Print and shaded views of the part. All mm, measured from the part's lowest x, y and z. Coordinates: 2 decimals unless noted, no trailing zeros. Loops run counter-clockwise (first coordinate to the right, second up) from the corner with the lowest first, then second, coordinate; pieces in that order, holes last.
1) Two-plate mould, pull along X, no slides. Class the marked faces 1, 2 and 3: +X half, -X half, draft (parallel to the pull), parting line (faces both ways), or undercut.
2) Saw through at C-C, the plane y = 5.25. Write the cut outline in (x, z), and give its area (3 significant figures).
3) Saw through at B-B, the plane x = 44. Write the cut outline in (y, z).
4) Wall check: line 1 along X through (y, z) = (8, 44); line 2 along X through (y, z) = (6.75, 62.5) (1 decimal); line 3 along X through (y, z) = (0.5, 25). Give the ranges that are in metal, low to high.
5) Pin check, flat tips, straight feed: pin 1 Ø3 at (y, z) = (6.5, 48) entering from -X; pin 2 Ø2.5 at (x, z) = (76.04, 62.5) entering from +Y; pin 3 Ø4 at (x, z) = (12.5, 14) entering from -Y; pin 4 Ø4 at (y, z) = (9.5, 66.5) entering from +X. Stop position of each tip, or through.
6) Saw through at D-D, the plane z = 62.5. Write the cut outline in (x, y).
7) Saw through at A-A, the plane z = 44. Write the cut outline in (x, y).
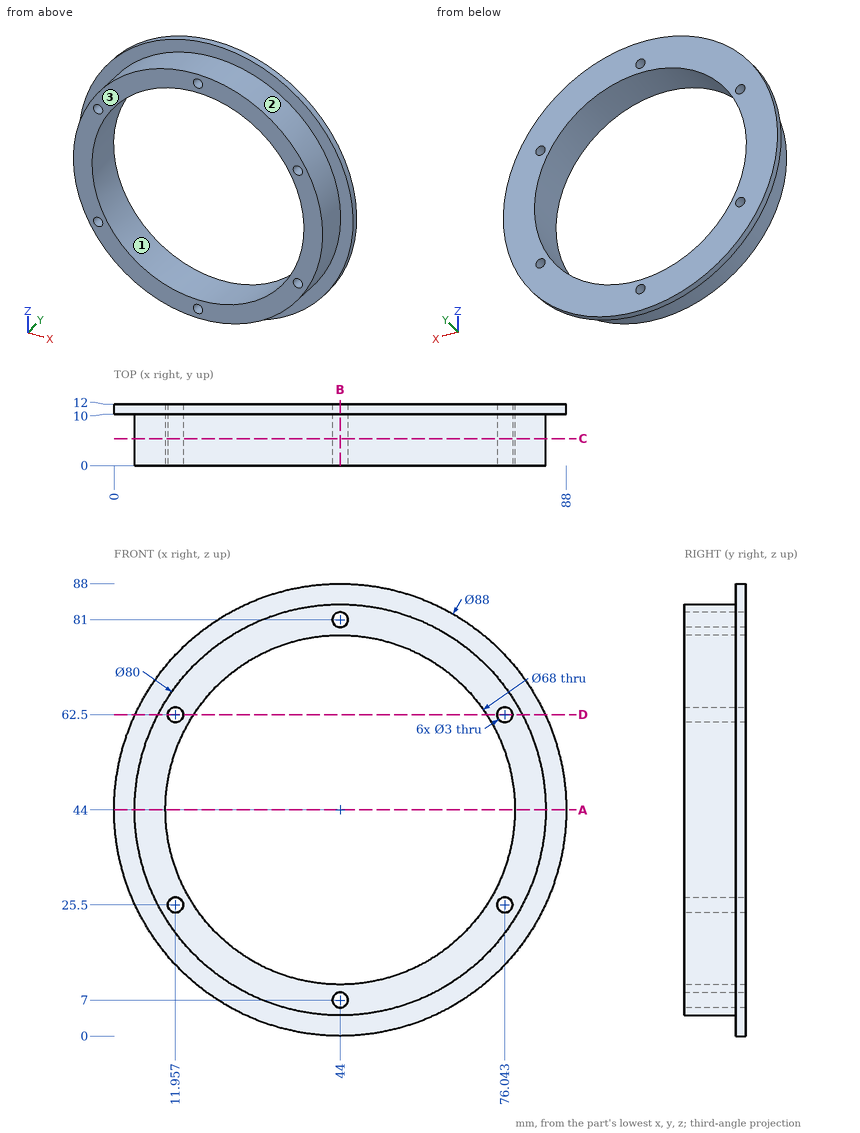
Data:
1. face 1: undercut
1. face 2: parting line
1. face 3: draft
2. outline: circle Ø80 at (44, 44); hole circle Ø68 at (44, 44); hole circle Ø3 at (11.96, 25.5); hole circle Ø3 at (11.96, 62.5); hole circle Ø3 at (44, 7); hole circle Ø3 at (44, 81); hole circle Ø3 at (76.04, 25.5); hole circle Ø3 at (76.04, 62.5)
2. area: 1,350 mm2
3. outline: (0, 4) - (10, 4) - (10, 0) - (12, 0) - (12, 5.5) - (0, 5.5) - close; (0, 8.5) - (12, 8.5) - (12, 10) - (0, 10) - close; (0, 78) - (12, 78) - (12, 79.5) - (0, 79.5) - close; (0, 82.5) - (12, 82.5) - (12, 88) - (10, 88) - (10, 84) - (0, 84) - close
4. line 1: x = 4 to 10, 78 to 84
4. line 2: x = 8.5 to 10.5, 13.5 to 15.5, 72.5 to 74.5, 77.5 to 79.5
4. line 3: x = 8.8 to 10.54, 13.37 to 15.8, 72.2 to 74.63, 77.46 to 79.2
5. pin 1: stops at x = 4.08
5. pin 2: passes through
5. pin 3: stops at y = 10
5. pin 4: stops at x = 82.9
6. outline: (4.08, 10) - (8.54, 10) - (8.54, 0) - (10.46, 0) - (10.46, 12) - (4.08, 12) - close; (13.46, 0) - (15.47, 0) - (15.47, 12) - (13.46, 12) - close; (72.53, 0) - (74.54, 0) - (74.54, 12) - (72.53, 12) - close; (77.54, 0) - (79.46, 0) - (79.46, 10) - (83.92, 10) - (83.92, 12) - (77.54, 12) - close
7. outline: (0, 10) - (4, 10) - (4, 0) - (10, 0) - (10, 12) - (0, 12) - close; (78, 0) - (84, 0) - (84, 10) - (88, 10) - (88, 12) - (78, 12) - close
